Drawing for the job (mm, zero at the part's lowest x, y, z). Round coordinates to 2 decimals unless told otherwise and drop trailing zeros. Loops run counter-clockwise (first coordinate to the right, second up) from the corner with the lowest first, then second, coordinate; pieces in that order, holes last. Notation, with made-up numbers: (85, -14.5) -> (106, -14.5) arc R26 ccw to (106, 24.5) -> close; hole circle Ø9 at (-19, 84). An arc over 180 degrees is marked (long way). Put each result on its own line as item: value. Start each with the question number.
Item 1: Cut at C-C, the plane x = 191.5. List the corners of the cut face in (y, z), plus the area to 3 significant figures.
Item 2: Drill centre lines: probe 1 along Z at (x, y) = (166.5, 136.5); probe 2 along Z at (x, y) = (142.5, 33); probe 3 along Y at (x, z) = (96, 145.5). Where is each one in solid material? Low to high. Write a range as [from, to].
Item 3: Cut at A-A, the plane y = 123.5. List the corners of the cut face in (x, z), plus the area to 3 significant figures.
Item 4: Cut at D-D, the plane z = 185.5. List the corners of the cut face in (x, y), plus the area to 3 significant figures.
Item 5: Flat gauge pins, fed straight in: pin 1 Ø10 at (y, z) = (183, 80) entering from +X; pin 2 Ø8 at (y, z) = (102.5, 43) entering from -X; pin 3 Ø10 at (x, z) = (127, 29) entering from +Y. Where does each tip first touch, or does it go through?
Item 6: Cut at B-B, the plane z = 162.5. List the corners of the cut face in (x, y), plus the area to 3 significant figures.
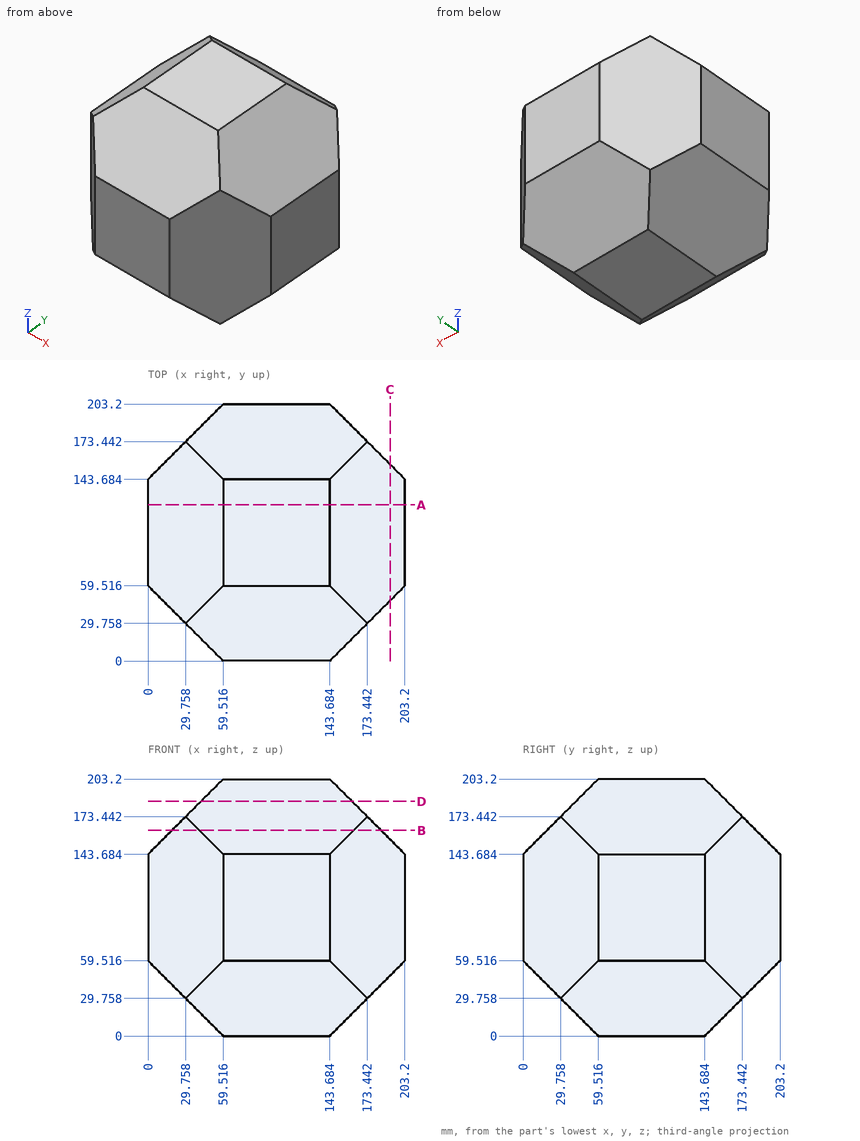
Reply:
1. outline: (47.82, 47.82) -> (155.38, 47.82) -> (155.38, 155.38) -> (47.82, 155.38) -> close
1. area: 11,600 mm^2
2. probe 1: z = [22.82, 180.38]
2. probe 2: z = [26.52, 176.68]
2. probe 3: y = [1.82, 201.38]
3. outline: (0, 59.52) -> (59.52, 0) -> (143.68, 0) -> (203.2, 59.52) -> (203.2, 143.68) -> (143.68, 203.2) -> (59.52, 203.2) -> (0, 143.68) -> close
3. area: 34,200 mm^2
4. outline: (41.82, 41.82) -> (161.38, 41.82) -> (161.38, 161.38) -> (41.82, 161.38) -> close
4. area: 14,300 mm^2
5. pin 1: stops at x = 168.88
5. pin 2: stops at x = 12.52
5. pin 3: stops at y = 177.68
6. outline: (18.82, 40.7) -> (40.7, 18.82) -> (162.5, 18.82) -> (184.38, 40.7) -> (184.38, 162.5) -> (162.5, 184.38) -> (40.7, 184.38) -> (18.82, 162.5) -> close
6. area: 26,500 mm^2
